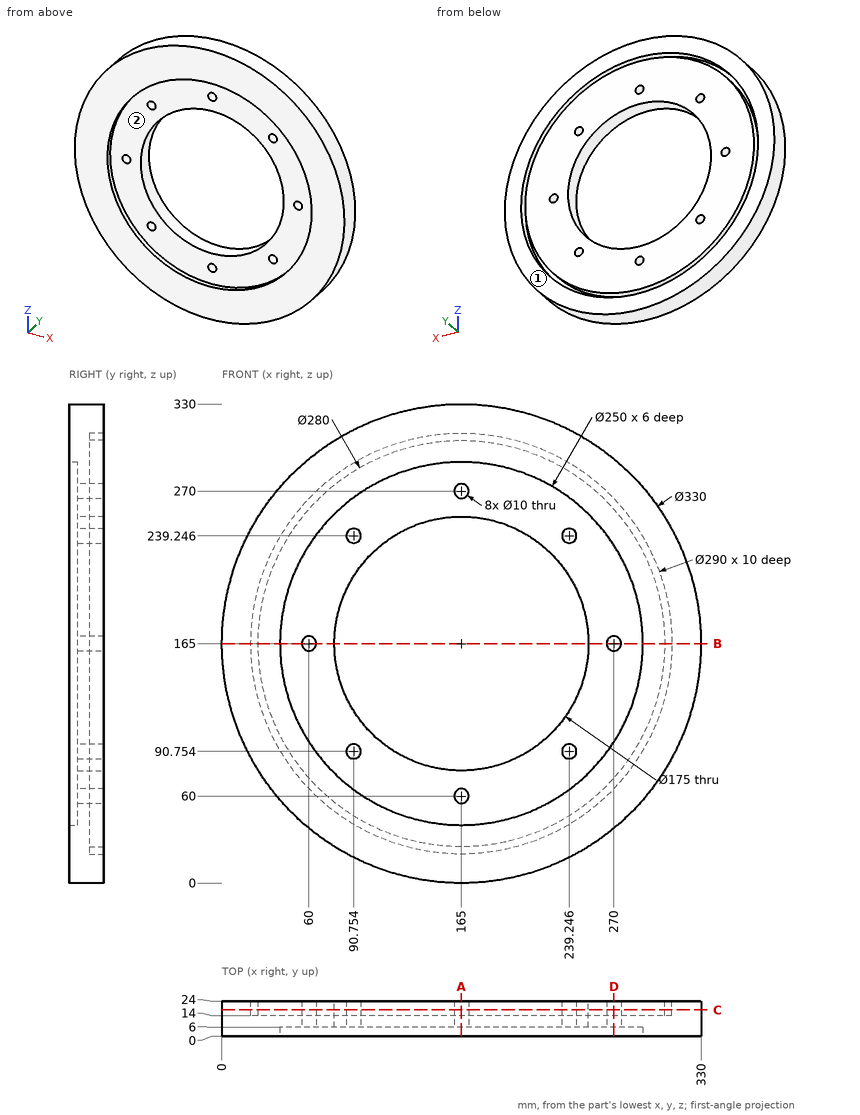
Geometry check sheet. Reference: drawing and pictorial views, mm from the part's lowest x, y, z. Round coordinates to 2 decimals unless told otherwise and drop trailing zeros. Loops run counter-clockwise (first coordinate to the right, second up) from the corner with the lowest first, then second, coordinate; pieces in that order, holes last. Notation, with made-up numbers: (-20, 7.25) -> (6, 7.25) arc R13 cw to (6, 18.25) -> close; hole circle Ø8 at (8.25, 48). An arc over 180 degrees is marked (long way). Use a Markdown table: item, result.
(1) Sectioned sample at D-D (x = 270). Enter the section's corners in (y, z).
Calculated:
| item | result |
|---|---|
| outline | (0, 37.72) -> (24, 37.72) -> (24, 65) -> (14, 65) -> (14, 72.4) -> (24, 72.4) -> (24, 160) -> (6, 160) -> (6, 97.18) -> (0, 97.18) -> close; (0, 232.82) -> (6, 232.82) -> (6, 170) -> (24, 170) -> (24, 257.6) -> (14, 257.6) -> (14, 265) -> (24, 265) -> (24, 292.28) -> (0, 292.28) -> close |
(2) Sectioned sample at C-C (y = 18). Give the number of separate pieces and of enclosed holes in the cut face, then the cut area to 3 significant figures.
Calculated:
| item | result |
|---|---|
| separate pieces | 2 |
| enclosed holes | 10 |
| area | 56,400 mm² |
(3) Sectioned sample at B-B (z = 165). Enter the section's corners in (x, y).
Calculated:
| item | result |
|---|---|
| outline | (0, 0) -> (40, 0) -> (40, 6) -> (55, 6) -> (55, 24) -> (25, 24) -> (25, 14) -> (20, 14) -> (20, 24) -> (0, 24) -> close; (65, 6) -> (77.5, 6) -> (77.5, 24) -> (65, 24) -> close; (252.5, 6) -> (265, 6) -> (265, 24) -> (252.5, 24) -> close; (275, 6) -> (290, 6) -> (290, 0) -> (330, 0) -> (330, 24) -> (310, 24) -> (310, 14) -> (305, 14) -> (305, 24) -> (275, 24) -> close |
(4) Mould release check, pull along X, two halves, no side actions. Record for the marked faces 1 and 2: released by +X, released by -X, zero draft, split by the parting line, or undercut.
Calculated:
| item | result |
|---|---|
| face 1 | zero draft |
| face 2 | undercut |
(5) Go/stop test with flat-tipped pins: P1, Ø8, axis at x = 60.5, y = 20.5, coming from the +Z side; P2, Ø5, axis at y = 20.5, z = 292, coming from the +X side; P3, Ø2, axis at x = 274, y = 17, coming from the +Z side. Record where each tip stops, or that it passes through.
Calculated:
| item | result |
|---|---|
| P1 | z = 295.86 |
| P2 | x = 273.28 |
| P3 | z = 289.74 |
(6) Sectioned sample at A-A (x = 165). Enter the section's corners in (y, z), then the cut area to 3 significant figures.
Calculated:
| item | result |
|---|---|
| outline | (0, 0) -> (24, 0) -> (24, 20) -> (14, 20) -> (14, 25) -> (24, 25) -> (24, 55) -> (6, 55) -> (6, 40) -> (0, 40) -> close; (0, 290) -> (6, 290) -> (6, 275) -> (24, 275) -> (24, 305) -> (14, 305) -> (14, 310) -> (24, 310) -> (24, 330) -> (0, 330) -> close; (6, 65) -> (24, 65) -> (24, 77.5) -> (6, 77.5) -> close; (6, 252.5) -> (24, 252.5) -> (24, 265) -> (6, 265) -> close |
| area | 2,810 mm² |
(7) Scan lines: probe 1 along X at (y, z) = (16.5, 165); probe 2 along Z at (x, y) = (179, 15.5) (1 decimal); probe 3 along X at (y, z) = (20.25, 132) (1 decimal). Record each from-to range of solid material in increasing order.
Calculated:
| item | result |
|---|---|
| probe 1 | 0 to 20, 25 to 55, 65 to 77.5, 252.5 to 265, 275 to 305, 310 to 330 |
| probe 2 | 0.6 to 20.7, 25.7 to 78.6, 251.4 to 304.3, 309.3 to 329.4 |
| probe 3 | 3.3 to 23.8, 28.9 to 84, 246 to 301.1, 306.2 to 326.7 |
